```python
from build123d import *

# Parameters (mm, degrees)
SKETCH1_W           = 16
SKETCH1_H           = 17
SKETCH1_R           = 4
BOSS_EXTRUDE1_DEPTH = 15
SKETCH2_W           = 5
SKETCH2_H           = 17
BOSS_EXTRUDE2_DEPTH = 16
SKETCH3_R           = 5.5
CUT_EXTRUDE3_DEPTH  = 16
BOSS_EXTRUDE5_DEPTH = 17
SKETCH5_R           = 1.25
CUT_EXTRUDE4_DEPTH  = 17
FILLET1_R           = 2
CHAMFER1_SIZE       = 0.5


with BuildPart() as part:
    # Sketch1 → Boss-Extrude1 (new body)
    with BuildSketch(Plane.XY):
        Rectangle(SKETCH1_W, SKETCH1_H)
        Circle(SKETCH1_R, mode=Mode.SUBTRACT)
    extrude(amount=BOSS_EXTRUDE1_DEPTH)

    # Sketch2 → Boss-Extrude2 (add)
    with BuildSketch(Plane.XY.offset(15)):
        with Locations((-5.5, 0)):
            Rectangle(SKETCH2_W, SKETCH2_H)
        with Locations((5.5, 0)):
            Rectangle(SKETCH2_W, SKETCH2_H)
    extrude(amount=BOSS_EXTRUDE2_DEPTH)

    # Sketch3 → Cut-Extrude3 (cut)
    with BuildSketch(Plane.ZY.offset(8)):
        with Locations((22.5, 0)):
            Circle(SKETCH3_R)
    extrude(amount=-CUT_EXTRUDE3_DEPTH, mode=Mode.SUBTRACT)

    # Sketch4 → Boss-Extrude5 (add, through all)
    with BuildSketch(Plane.XZ.offset(8.5)):
        Polygon((-3, 19), (-3, 15), (0, 15), (3, 15), (3, 19), (0, 17), align=None)
    extrude(amount=-BOSS_EXTRUDE5_DEPTH)

    # Sketch5 → Cut-Extrude4 (cut, through all)
    with BuildSketch(Plane(origin=(0, 0, 15), x_dir=(-1, 0, 0), z_dir=(0, 0, -1))):
        Circle(SKETCH5_R)
    extrude(amount=-CUT_EXTRUDE4_DEPTH, mode=Mode.SUBTRACT)

    # Fillet1
    fillet1_edges = [part.edges().sort_by_distance(p)[0] for p in [
        (-3, 8.5, 25),
        (-3, -8.5, 25),
        (-5.5, 8.5, 31),
        (-8, 0, 31),
        (-5.5, -8.5, 31),
        (-3, 0, 31),
        (3, 8.5, 25),
        (3, -8.5, 25),
        (5.5, 8.5, 31),
        (3, 0, 31),
        (5.5, -8.5, 31),
        (8, 0, 31),
        (0, -8.5, 0),
        (-8, 0, 0),
        (0, 8.5, 0),
        (8, 0, 0),
        (-1.5, 8.5, 18),
        (1.5, 8.5, 18),
        (1.5, -8.5, 18),
        (-1.5, -8.5, 18),
        (8, -8.5, 15.5),
        (-8, -8.5, 15.5),
        (-8, 8.5, 15.5),
        (8, 8.5, 15.5),
    ]]
    fillet(fillet1_edges, radius=FILLET1_R)

    # Chamfer1
    chamfer1_edges = [part.edges().sort_by_distance(p)[0] for p in [
        (-4, 0, 0),
        (8, 0, 17),
        (-8, 0, 17),
    ]]
    chamfer(chamfer1_edges, length=CHAMFER1_SIZE)


solid = part.part
```
Check sheet for the modelled part. Datum: model origin and axes. Units: mm. A direction names the side the tool comes from. Round coordinates to 2 decimals unless told otherwise and drop trailing zeros. Write each loop counter-clockwise with the first axis right and the second up, starting at its lowest first coordinate (ties: lowest second). Pieces come first, ordered by that corner, then holes. Notation, with made-up numbers: (13, 55.5) -> (51, 55.5) arc R20 cw to (51, 93.5) -> close; hole circle Ø5 at (23, 70). An arc over 180 degrees is marked (long way). Put each result on its own line as item: value.
(1) Go/stop test with flat-tipped pins: pin 1 Ø1 at (y, z) = (-1, 18.5) entering from -X; pin 2 Ø2.5 at (x, y) = (0.5, -2) entering from -Z; pin 3 Ø1 at (y, z) = (1, 18.5) entering from +X; pin 4 Ø6 at (y, z) = (-3, 21) entering from +X. Record where each tip stops, or that it passes through.
Values found:
pin 1: stops at x = -3
pin 2: stops at z = 15
pin 3: stops at x = 3
pin 4: stops at x = 8
(2) Tool access check on faces 4 (the face through (5.22, -2.11, 27.58)), 5 (the face through (-3.57, 7.9, 23.54)), 6 (the face through (-3.57, 0.09, 30.4)), 7 (the face through (-1, -1, 15)). Record the directions out of +Z, -Z, +X, -X, +Y, -Y that give a thin tool (end or side, any length) a straight path to the whole face; none if there is none.
Values found:
face 4: +X
face 5: +Z, +Y
face 6: +Z, +Y, -Y
face 7: -Z
(3) Sectioned sample at A-A (z = 22.5). Enter the section's corners in (x, y).
Values found:
outline: (-8, -6.5) arc R2 ccw to (-6, -8.5) -> (-5, -8.5) arc R2 ccw to (-3, -6.5) -> (-3, -5.5) -> (-7.5, -5.5) -> (-8, -6) -> close; (-8, 6) -> (-7.5, 5.5) -> (-3, 5.5) -> (-3, 6.5) arc R2 ccw to (-5, 8.5) -> (-6, 8.5) arc R2 ccw to (-8, 6.5) -> close; (3, -6.5) arc R2 ccw to (5, -8.5) -> (6, -8.5) arc R2 ccw to (8, -6.5) -> (8, -6) -> (7.5, -5.5) -> (3, -5.5) -> close; (3, 5.5) -> (7.5, 5.5) -> (8, 6) -> (8, 6.5) arc R2 ccw to (6, 8.5) -> (5, 8.5) arc R2 ccw to (3, 6.5) -> close
(4) Sectioned sample at C-C (y = -2.5). Count the separate pieces of the cut face and the enclosed holes in it, plus the area to 3 significant figures.
Values found:
separate pieces: 3
enclosed holes: 0
area: 220 mm^2
(5) Mould release check, pull along Z, two halves, no side actions. Record for faces 1 (the face through (7.4, 7.93, 15.31)), 2 (the face through (-5.28, -2.11, 27.58)), 3 (the face through (5.51, -7.93, 30.4)): released by +Z, released by -Z, zero draft, split by the parting line, or undercut.
Values found:
face 1: zero draft
face 2: undercut
face 3: released by +Z
(6) Material ranges on line 1 (X direction, y = 0, z = 16.25); line 2 (Z direction, x = 5.6, y = 0); line 3 (Y direction, x = -5.95, z = 22.5), recorded low to high.
Values found:
line 1: x = -8 to -1.25, 1.25 to 8
line 2: z = 0 to 17, 28 to 31
line 3: y = -8.5 to -5.5, 5.5 to 8.5
(7) Sectioned sample at B-B (z = 10.5). Enter the section's corners in (x, y), plus the area to 3 significant figures.
Values found:
outline: (-8, -6.5) arc R2 ccw to (-6, -8.5) -> (6, -8.5) arc R2 ccw to (8, -6.5) -> (8, 6.5) arc R2 ccw to (6, 8.5) -> (-6, 8.5) arc R2 ccw to (-8, 6.5) -> close; hole circle Ø8 at (0, 0)
area: 218 mm^2
